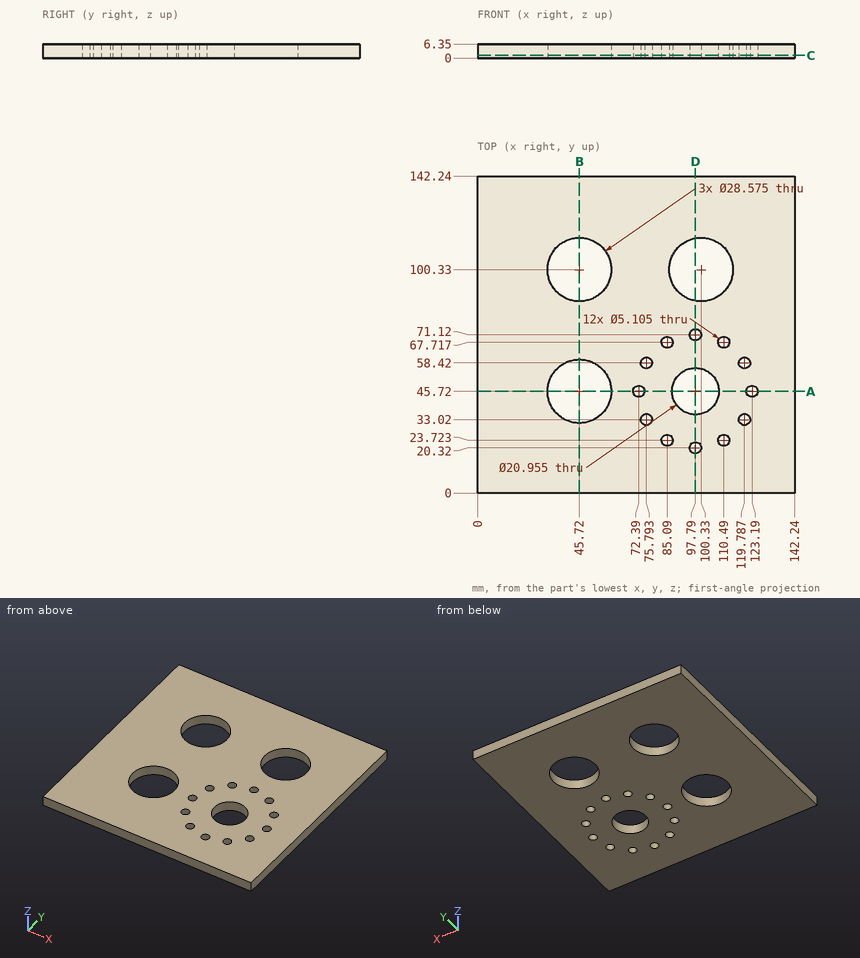
Print and shaded views of the part. All mm, measured from the part's lowest x, y and z. Round coordinates to 2 decimals unless told otherwise and drop trailing zeros. Write each loop counter-clockwise with the first axis right and the second up, starting at its lowest first coordinate (ties: lowest second). Pieces come first, ordered by that corner, then holes. Notation, with made-up numbers: M -3,-16.5 L 17,-16.5 A27 cw 17,1.5 Z; hole C 34,45 d5. An arc over 180 degrees is marked long. Use a Markdown table: item, result. Add a question column.
1. Drill centre lines: probe 1 along Y at (x, z) = (85.09, 3) (1 decimal); probe 2 along X at (y, z) = (45.72, 3); probe 3 along X at (y, z) = (20.32, 4.75). Where is each one in solid material? Low to high.
2. Slice it at A-A on y = 45.72. Give the cut face in (x, z).
3. Slice it at C-C on z = 1.25. Give the number of separate pieces and of enclosed holes in the cut face, then the cut area to 3 significant figures.
4. Flat gauge pin, fed straight in: P1, Ø6, axis at x = 97.79, y = 71.12, coming from the -Z side. Where does the tip first touch, or does it go through?
5. Slice it at B-B on x = 45.72. Give the cut face in (y, z), then the cut area to 3 significant figures.
6. Slice it at D-D on x = 97.79. Give the cut face in (y, z).
Reply:
| question | item | result |
|---|---|---|
| 1 | probe 1 | y = 0 to 21.2, 26.3 to 65.2, 70.3 to 142.2 |
| 1 | probe 2 | x = 0 to 31.43, 60.01 to 69.84, 74.94 to 87.31, 108.27 to 120.64, 125.74 to 142.24 |
| 1 | probe 3 | x = 0 to 95.24, 100.34 to 142.24 |
| 2 | outline | M 0,0 L 31.43,0 L 31.43,6.35 L 0,6.35 Z; M 60.01,0 L 69.84,0 L 69.84,6.35 L 60.01,6.35 Z; M 74.94,0 L 87.31,0 L 87.31,6.35 L 74.94,6.35 Z; M 108.27,0 L 120.64,0 L 120.64,6.35 L 108.27,6.35 Z; M 125.74,0 L 142.24,0 L 142.24,6.35 L 125.74,6.35 Z |
| 3 | separate pieces | 1 |
| 3 | enclosed holes | 16 |
| 3 | area | 17,700 mm^2 |
| 4 | P1 | stops at z = 0 |
| 5 | outline | M 0,0 L 31.43,0 L 31.43,6.35 L 0,6.35 Z; M 60.01,0 L 86.04,0 L 86.04,6.35 L 60.01,6.35 Z; M 114.62,0 L 142.24,0 L 142.24,6.35 L 114.62,6.35 Z |
| 5 | area | 540 mm^2 |
| 6 | outline | M 0,0 L 17.77,0 L 17.77,6.35 L 0,6.35 Z; M 22.87,0 L 35.24,0 L 35.24,6.35 L 22.87,6.35 Z; M 56.2,0 L 68.57,0 L 68.57,6.35 L 56.2,6.35 Z; M 73.67,0 L 86.27,0 L 86.27,6.35 L 73.67,6.35 Z; M 114.39,0 L 142.24,0 L 142.24,6.35 L 114.39,6.35 Z |
